Can you work these out from the model? Positions are in its coordinate system, mm. Coordinates: 2 decimals unless noted, no trailing zeros. Order: outer loops, then holes, each group sorted by start corner. A loop starts at its lowest first (then second) coordinate and runs counter-clockwise, first axis right, second up. Notation, with made-up numbers: (23.5, -13.75) -> (32.5, -13.75) arc R33 cw to (32.5, 22.25) -> close; hole circle Ø10 at (76, 17). An arc over 180 degrees is marked (long way). Answer in a Markdown table with one row per item. Add a question column.
1. Imagine slicing it at B-B on x = 7. Write out the boundary of the cut face in (y, z), plus the area to 3 significant figures.
2. Imagine slicing it at A-A on z = 0.1. Write out the boundary of the cut face in (x, y), plus the area to 3 significant figures.
3. Imagine slicing it at D-D on x = 3. Write out the boundary of the cut face in (y, z).
4. We'd pull the mould along X, two halves only. Please class faces 1 (the face through (4.5, 3.4, 0.56)), 2 (the face through (13.082, 3.032, 0.276)), 3 (the face through (14.746, 2.209, 0.276)): pulls with the +X half, pulls with the -X half, needs draft (parallel to the pull), parting line crosses it, or undercut.
5. If I drill on line 1 along X through (y, z) = (2.55, 0.2); line 2 along X through (y, z) = (2.7, 0.45); line 3 along Y through (x, z) = (8.25, 0.1), over which ranges is the centre line in solid material (lowest first)? Write a range as [from, to].
6. Imagine slicing it at C-C on y = 0.6. Write out the boundary of the cut face in (x, z), plus the area to 3 significant figures.
from build123d import *

# Parameters (mm, degrees)
F0_W     = 0.5
F0_H     = 0.3
F0_R     = 0.75
F1_DEPTH = 0.56


with BuildPart() as f1:
    # F0 (on Top) → F1 (new body)
    with BuildSketch(Plane.XY):
        with BuildLine():
            Line((14, 4), (0, 4))
            Line((0, 4), (-2, 4))
            Line((-2, 4), (-2, 0))
            Line((-2, 0), (0, 0))
            Line((0, 0), (14.132164, 1.884288))
            ThreePointArc((14.132164, 1.884288), (14.752384, 2.216792), (15, 2.875516))
            Line((15, 2.875516), (15, 3))
            ThreePointArc((15, 3), (14.707107, 3.707107), (14, 4))
        make_face()
        with Locations((-0.55, 0.95)):
            Rectangle(F0_W, F0_H, mode=Mode.SUBTRACT)
        with Locations((1.981743, 2.249582)):
            Circle(F0_R, mode=Mode.SUBTRACT)
        with Locations((4.578013, 2.3888)):
            Circle(F0_R, mode=Mode.SUBTRACT)
        with Locations((-0.55, 3.05)):
            Rectangle(F0_W, F0_H, mode=Mode.SUBTRACT)
        with Locations((7.174283, 2.528018)):
            Circle(F0_R, mode=Mode.SUBTRACT)
        with Locations((9.770553, 2.667237)):
            Circle(F0_R, mode=Mode.SUBTRACT)
        with Locations((12.366823, 2.806455)):
            Circle(F0_R, mode=Mode.SUBTRACT)
    extrude(amount=F1_DEPTH)


solid = f1.part
Answers follow:
| question | item | result |
|---|---|---|
| 1 | outline | (0.93, 0) -> (1.8, 0) -> (1.8, 0.56) -> (0.93, 0.56) -> close; (3.26, 0) -> (4, 0) -> (4, 0.56) -> (3.26, 0.56) -> close |
| 1 | area | 0.900 mm² |
| 2 | outline | (-2, 0) -> (0, 0) -> (14.13, 1.88) arc R1 ccw to (15, 2.88) -> (15, 3) arc R1 ccw to (14, 4) -> (-2, 4) -> close; hole (-0.8, 0.8) -> (-0.3, 0.8) -> (-0.3, 1.1) -> (-0.8, 1.1) -> close; hole (-0.8, 2.9) -> (-0.3, 2.9) -> (-0.3, 3.2) -> (-0.8, 3.2) -> close; hole circle Ø1.5 at (1.98, 2.25); hole circle Ø1.5 at (4.58, 2.39); hole circle Ø1.5 at (7.17, 2.53); hole circle Ø1.5 at (9.77, 2.67); hole circle Ø1.5 at (12.37, 2.81) |
| 2 | area | 43.5 mm² |
| 3 | outline | (0.4, 0) -> (4, 0) -> (4, 0.56) -> (0.4, 0.56) -> close |
| 4 | face 1 | needs draft |
| 4 | face 2 | undercut |
| 4 | face 3 | pulls with the +X half |
| 5 | line 1 | x = [-2, 1.29], [2.67, 3.85], [5.31, 6.42], [7.92, 9.03], [10.51, 11.66], [13.07, 14.95] |
| 5 | line 2 | x = [-2, 1.38], [2.58, 3.9], [5.26, 6.44], [7.9, 9.02], [10.52, 11.62], [13.11, 14.98] |
| 5 | line 3 | y = [1.1, 4] |
| 6 | outline | (-2, 0) -> (4.5, 0) -> (4.5, 0.56) -> (-2, 0.56) -> close |
| 6 | area | 3.64 mm² |
